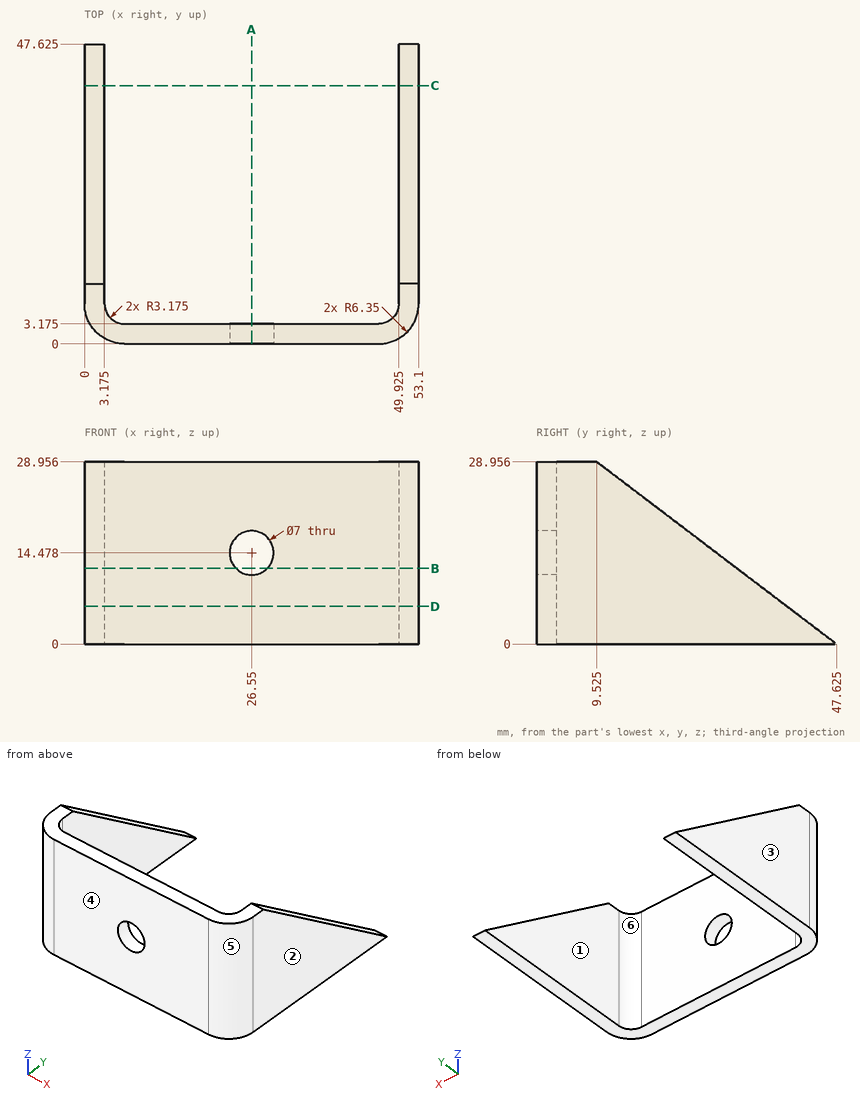
Check sheet for the drawn part. Datum: minimum x, y, z corner. Units: mm. A direction names the side the tool comes from. Round coordinates to 2 decimals unless told otherwise and drop trailing zeros. Order: outer loops, then holes, each group sorted by start corner. A loop starts at its lowest first (then second) coordinate and runs counter-clockwise, first axis right, second up. Notation, with made-up numbers: (-31.75, -8) -> (-4.75, -8) arc R18 cw to (-4.75, 24) -> close; hole circle Ø8 at (63, 43.5). An arc over 180 degrees is marked (long way). Put each result on its own line as item: value.
1) Mould release check, pull along X, two halves, no side actions. Record for the marked faces 3, 4, 5 and 6: +X half, -X half, draft (parallel to the pull), parting line (faces both ways), or undercut.
Final values:
face 3: -X half
face 4: draft
face 5: +X half
face 6: undercut
2) Section check B-B (z = 12). Record the cut outline in (x, y) (3 decimals), then the cut area to 3 significant figures.
Final values:
outline: (0, 6.35) arc R6.35 ccw to (6.35, 0) -> (24.078, 0) -> (24.078, 3.175) -> (6.35, 3.175) arc R3.175 cw to (3.175, 6.35) -> (3.175, 31.836) -> (0, 31.836) -> close; (29.022, 0) -> (46.75, 0) arc R6.35 ccw to (53.1, 6.35) -> (53.1, 31.836) -> (49.925, 31.836) -> (49.925, 6.35) arc R3.175 cw to (46.75, 3.175) -> (29.022, 3.175) -> close
area: 322 mm^2
3) Section check A-A (x = 26.55). Record the cut outline in (y, z) (3 decimals), then the cut area to 3 significant figures.
Final values:
outline: (0, 0) -> (3.175, 0) -> (3.175, 10.978) -> (0, 10.978) -> close; (0, 17.978) -> (3.175, 17.978) -> (3.175, 28.956) -> (0, 28.956) -> close
area: 69.7 mm^2
4) Set-up check for the marked faces 1 and 2: record each of +Z, -Z, +X, -X, +Y, -Y from which the full face is reachable in a straight line by a thin tool's end or side.
Final values:
face 1: +Z, -Z, +Y
face 2: +Z, -Z, +X, +Y, -Y
5) Section check C-C (y = 41). Record the cut outline in (x, z) (3 decimals).
Final values:
outline: (0, 0) -> (3.175, 0) -> (3.175, 5.035) -> (0, 5.035) -> close; (49.925, 0) -> (53.1, 0) -> (53.1, 5.035) -> (49.925, 5.035) -> close
6) Section check D-D (z = 6). Record the cut outline in (x, y) (3 decimals).
Final values:
outline: (0, 6.35) arc R6.35 ccw to (6.35, 0) -> (46.75, 0) arc R6.35 ccw to (53.1, 6.35) -> (53.1, 39.73) -> (49.925, 39.73) -> (49.925, 6.35) arc R3.175 cw to (46.75, 3.175) -> (6.35, 3.175) arc R3.175 cw to (3.175, 6.35) -> (3.175, 39.73) -> (0, 39.73) -> close
7) Material ranges on line 1 (X direction, y = 8, z = 27) (3 decimals); line 2 (Z direction, x = 26.55, y = 1.95); line 3 (Y direction, x = 9.5, z = 13.25) (3 decimals), recorded low to high.
Final values:
line 1: x = 0 to 3.175, 49.925 to 53.1
line 2: z = 0 to 10.98, 17.98 to 28.96
line 3: y = 0 to 3.175
8) Depth check by flat-ended pin: pin 1 (1.5 mm diameter, centred on x = 8, z = 3, fed in from +Y) (3 decimals); pin 2 (4 mm diameter, centred on x = 27, z = 15.5, fed in from +Y); pin 3 (6 mm diameter, centred on y = 13.5, z = 13.5, fed in from -X). Enter the tip coordinate at first touch or a pass-through.
Final values:
pin 1: stops at y = 3.175
pin 2: passes through
pin 3: stops at x = 0
